from build123d import *

# Parameters (mm, degrees)
F3_DEPTH     = 2.95
F4_T2_ANGLE  = 64.8878433285
F4_T4_ANGLE  = 64.8878433285
F4_S9_R      = 3.95
F4_T10_DEPTH = 8
F4_S15_R     = 3.95
F4_T16_DEPTH = 8
F5_R         = 0.2


# Not quite as in the source:
# - a fillet or chamfer that OpenCascade refuses, or shapes differently, is made with other operations: its cross-section is extruded or revolved along the edge and cut away or added


with BuildPart() as f1:
    # F0 (on Front) → F1 (revolve)
    with BuildSketch(Plane.XZ):
        Polygon((-11.75, 0), (0, 0), (0, 20.9), (-4.85, 20.9), (-4.85, 16.6), (-3.95, 16.6), (-3.95, 14.1), (-4.85, 14.1), (-4.85, 9.2), (-11.8, 9.2), (-11.8, 6.25), (-9.5, 6.25), (-9.5, 2.95), (-11.75, 2.95), align=None)
    revolve(axis=Axis((0, 0, 10.45), (0, 0, -1)))

    # F2 (on face) → F3 (cut, through all)
    with BuildSketch(Plane(origin=(0, 0, 0), x_dir=(1, 0, 0), z_dir=(0, 0, -1))):
        with BuildLine():
            Line((-4, -11.048189897), (-4, 11.048189897))
            ThreePointArc((-4, 11.048189897), (-11.75, 0), (-4, -11.048189897))
        make_face()
        with BuildLine():
            ThreePointArc((11.75, 0), (9.6193165038, 6.7476847881), (4, 11.048189897))
            Line((4, 11.048189897), (4, -11.048189897))
            ThreePointArc((4, -11.048189897), (9.6193165038, -6.7476847881), (11.75, 0))
        make_face()
    extrude(amount=-F3_DEPTH, mode=Mode.SUBTRACT)

    # F4: chamfer of 1 on 4 edges, made by hand

    # F4_s1 → F4_t2 (revolve, cut)
    with BuildSketch(Plane(origin=(0, 0, 0), x_dir=(0, 0, 1), z_dir=(0.8439169246, 0.5364738804, 0))):
        Polygon((0, 10.75), (1, 11.75), (0, 11.75), align=None)
    revolve(axis=Axis((0, 0, 0), (0, 0, -1)), revolution_arc=F4_T2_ANGLE, mode=Mode.SUBTRACT)

    # F4_s3 → F4_t4 (revolve, cut)
    with BuildSketch(Plane(origin=(0, 0, 0), x_dir=(0, 0, 1), z_dir=(-0.8439169246, -0.5364738804, 0))):
        Polygon((0, 10.75), (1, 11.75), (0, 11.75), align=None)
    revolve(axis=Axis((0, 0, 0), (0, 0, -1)), revolution_arc=F4_T4_ANGLE, mode=Mode.SUBTRACT)


with BuildPart() as f4_tool6:
    # F4_s7 → F4_t8 (revolve)
    with BuildSketch(Plane.XZ):
        Polygon((-3.85, 16.6), (-4.85, 17.6), (-4.85, 16.6), align=None)
    revolve(axis=Axis((0, 0, 16.6), (0, 0, -1)))

    # F4_s9 → F4_t10 (cut, symmetric)
    with BuildSketch(Plane.XY.offset(17.1)):
        Circle(F4_S9_R)
    extrude(amount=F4_T10_DEPTH, both=True, mode=Mode.SUBTRACT)


with BuildPart() as f1_1:
    add(f1.part)

    # F4_t5: cut F4_tool6
    add(f4_tool6.part, mode=Mode.SUBTRACT)


with BuildPart() as f4_tool12:
    # F4_s13 → F4_t14 (revolve)
    with BuildSketch(Plane.XZ):
        Polygon((-4.85, 13.1), (-3.85, 14.1), (-4.85, 14.1), align=None)
    revolve(axis=Axis((0, 0, 14.1), (0, 0, -1)))

    # F4_s15 → F4_t16 (cut, symmetric)
    with BuildSketch(Plane.XY.offset(13.6)):
        Circle(F4_S15_R)
    extrude(amount=F4_T16_DEPTH, both=True, mode=Mode.SUBTRACT)


with BuildPart() as f1_2:
    add(f1_1.part)

    # F4_t11: cut F4_tool12
    add(f4_tool12.part, mode=Mode.SUBTRACT)

    # F5
    f5_edges = [f1_2.edges().sort_by_distance(p)[0] for p in [
        (4.85, 0, 20.9),
    ]]
    fillet(f5_edges, radius=F5_R)


solid = f1_2.part
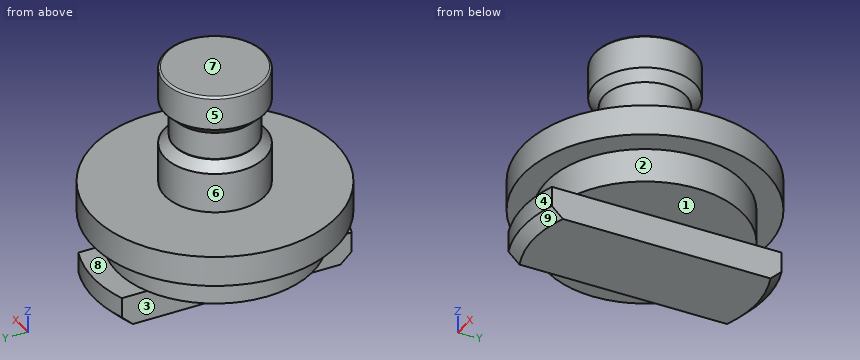
The listing builds one solid part. Answer for the finished solid, in the listing's coordinates (mm). Face numbers are marked on the shaded views. A direction names the side the tool comes from. Give positions to 0.01 mm unless a question says otherwise; leave off trailing zeros. Order: outer loops, then holes, each group sorted by start corner. A loop starts at its lowest first (then second) coordinate and runs counter-clockwise, first axis right, second up. Notation, with made-up numbers: (-15, 57.5) -> (41, 57.5) arc R17 cw to (41, 72.5) -> close; hole circle Ø8 at (74, 73). An arc over 180 degrees is marked (long way). Put each result on its own line as item: value.
Item 1: A cutting plane is placed at A-A on x = 0. Give the vertices of the cut face in (y, z), plus the area to 3 significant figures.
Established:
outline: (-11.8, 6.25) -> (-9.5, 6.25) -> (-9.5, 2.95) -> (-11.75, 2.95) -> (-11.75, 1) -> (-10.75, 0) -> (10.75, 0) -> (11.75, 1) -> (11.75, 2.95) -> (9.5, 2.95) -> (9.5, 6.25) -> (11.8, 6.25) -> (11.8, 9.2) -> (4.85, 9.2) -> (4.85, 13.1) -> (3.95, 14) -> (3.95, 16.7) -> (4.85, 17.6) -> (4.85, 20.7) arc R0.2 ccw to (4.65, 20.9) -> (-4.65, 20.9) arc R0.2 ccw to (-4.85, 20.7) -> (-4.85, 17.6) -> (-3.95, 16.7) -> (-3.95, 14) -> (-4.85, 13.1) -> (-4.85, 9.2) -> (-11.8, 9.2) -> close
area: 308 mm^2
Item 2: Given P1, Ø3, axis at y = 2.5, z = 2, coming from the -X side; P2, Ø5, axis at y = 6.5, z = 10, coming from the -X side; P3, Ø1, axis at x = -1, z = 16.5, coming from the -Y side, each flat-ended and moving along its own axis, determine where each tip first touches the part or whether it passes through.
Established:
P1: stops at x = -9.41
P2: stops at x = -11.05
P3: stops at y = -4.14
Item 3: A cutting plane is placed at D-D on x = -8.75. Give the vertices of the cut face in (y, z).
Established:
outline: (-7.92, 6.25) -> (-3.7, 6.25) -> (-3.7, 2.95) -> (3.7, 2.95) -> (3.7, 6.25) -> (7.92, 6.25) -> (7.92, 9.2) -> (-7.92, 9.2) -> close
Item 4: A cutting plane is placed at C-C on x = 6.5. Give the vertices of the cut face in (y, z).
Established:
outline: (-9.85, 6.25) -> (-6.93, 6.25) -> (-6.93, 2.95) -> (6.93, 2.95) -> (6.93, 6.25) -> (9.85, 6.25) -> (9.85, 9.2) -> (-9.85, 9.2) -> close
Item 5: For a pull along Z with two mould halves and no side action, classify the marked faces 6, 7, 8 and 9 as released by +Z, released by -Z, zero draft, split by the parting line, or undercut.
Established:
face 6: zero draft
face 7: released by +Z
face 8: undercut
face 9: released by -Z
Item 6: Straight lines are drawn through the part: line 1 (Z direction, x = 7.5, y = 8); line 2 (X direction, y = 4, z = 1); line 3 (Z direction, x = -3.5, y = 3.75). For each, find the intervals that lie inside material, in ascending order.
Established:
line 1: z = 6.25 to 9.2
line 2: x = -4 to 4
line 3: z = 0 to 9.2
Item 7: A cutting plane is placed at B-B on z = 8.25. Give the vertices of the cut face in (x, y), plus the area to 3 significant figures.
Established:
outline: circle Ø23.6 at (0, 0)
area: 437 mm^2
Item 8: For the marked faces 1, 2, 3, 4 and 5, determine the directions among +Z, -Z, +X, -X, +Y, -Y from which every point of the face is accessible in a straight line to the end or side of a thin tool.
Established:
face 1: -Z, +X, +Y, -Y
face 2: none
face 3: -Z, -X, +Y, -Y
face 4: -Z, -Y
face 5: +Z
